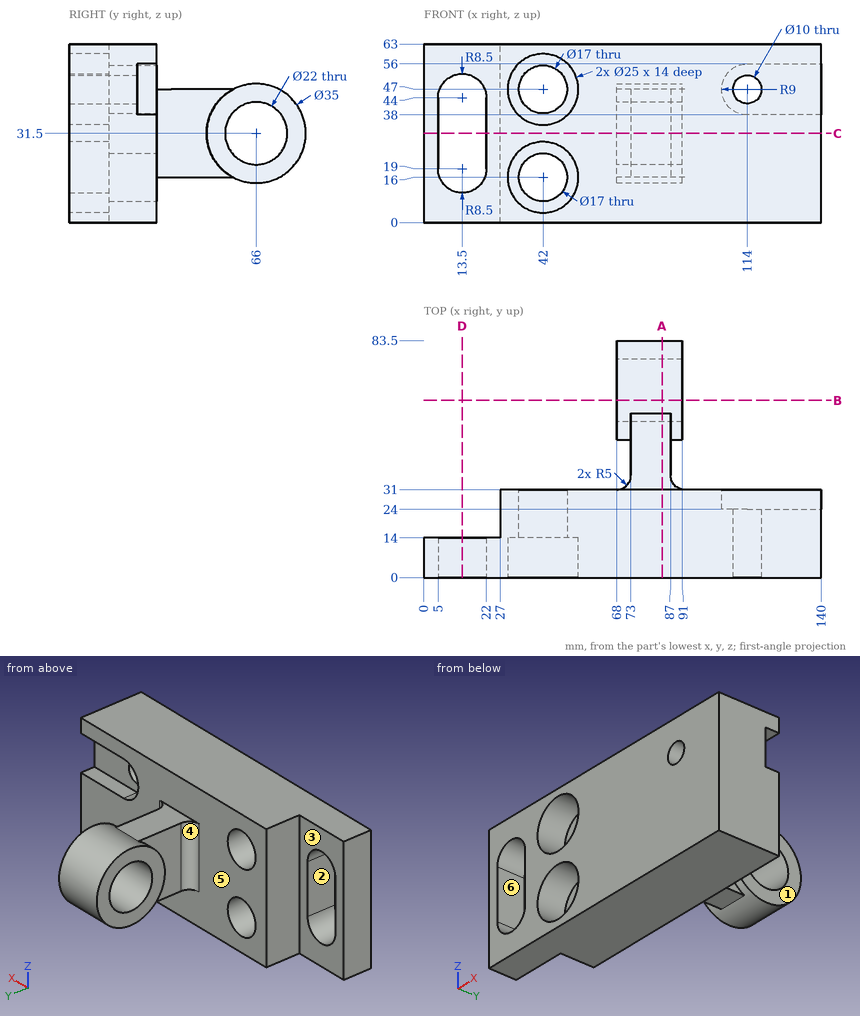
Here's the drawing with two shaded views (mm, measured from the low corner). I have some questions. A direction names the side the tool comes from. Give positions to 0.01 mm unless a question says otherwise; leave off trailing zeros. Loops run counter-clockwise (first coordinate to the right, second up) from the corner with the lowest first, then second, coordinate; pieces in that order, holes last. Notation, with made-up numbers: (-1, 32.25) - (30, 32.25) arc R17 cw to (30, 57.25) - close; hole circle Ø6 at (35, 40). An arc over 180 degrees is marked (long way). One line per item, written item: value.
(1) If we mould it in two halves opening along X, with no side actions, what happens to the marked faces 4, 5 and 6? For each: released by +X, released by -X, zero draft, split by the parting line, or undercut.
Verdict:
face 4: released by -X
face 5: zero draft
face 6: undercut
(2) On a 3-axis mill with a long thin cutter (end or side, diameter ignored), from which of +Z, -Z, +X, -X, +Y, -Y can I reach the whole of each face in a straight line? I mean the marked faces 1, 2 and 3. Say none if no direction works.
Verdict:
face 1: +Z, -Z, +X, +Y
face 2: +Y, -Y
face 3: +Z, -Z, -X, +Y
(3) I'm going to push flat-ended pins straight in: pin 1 (8 mm diameter, centred on y = 37, z = 46.5, fed in from -X); pin 2 (19 mm diameter, centred on x = 89, z = 44, fed in from +Y); pin 3 (17.5 mm diameter, centred on y = 50.5, z = 30.5, fed in from +X). Where does each tip first touch, or does it pass through?
Verdict:
pin 1: x = 72
pin 2: y = 83.24
pin 3: x = 91
(4) If we section it at B-B, the plane y = 62.5: List the corners of the cut face in (x, z) for me, plus the area to 3 significant figures.
Verdict:
outline: (68, 14.35) - (91, 14.35) - (91, 21.07) - (68, 21.07) - close; (68, 41.93) - (91, 41.93) - (91, 48.65) - (68, 48.65) - close
area: 309 mm^2
(5) If we section it at A-A, the plane x = 84: List the corners of the cut face in (y, z) for me.
Verdict:
outline: (0, 0) - (31, 0) - (31, 16) - (57.88, 16) arc R17.5 ccw (long way) to (57.88, 47) - (31, 47) - (31, 63) - (0, 63) - close; hole circle Ø22 at (66, 31.5)
(6) I need wall thicknesses on line 1 along Y through (x, z) = (74, 31); line 2 along X through (y, z) = (19.5, 16); line 3 along Z through (x, y) = (42, 22). Which ranges of each line are inside material? Lowest first, please.
Verdict:
line 1: 0 to 55.01, 76.99 to 83.49
line 2: 27 to 33.5, 50.5 to 140
line 3: 0 to 7.5, 24.5 to 38.5, 55.5 to 63
(7) If we section it at D-D, the plane x = 13.5: List the corners of the cut face in (y, z) for me, plus the area to 3 significant figures.
Verdict:
outline: (0, 0) - (14, 0) - (14, 10.5) - (0, 10.5) - close; (0, 52.5) - (14, 52.5) - (14, 63) - (0, 63) - close
area: 294 mm^2
(8) If we section it at C-C, the plane z = 31.5: List the corners of the cut face in (x, y) for me.
Verdict:
outline: (0, 0) - (5, 0) - (5, 14) - (0, 14) - close; (22, 0) - (140, 0) - (140, 31) - (92, 31) arc R5 cw to (87, 36) - (87, 48.5) - (91, 48.5) - (91, 55) - (68, 55) - (68, 48.5) - (73, 48.5) - (73, 36) arc R5 cw to (68, 31) - (27, 31) - (27, 14) - (22, 14) - close; (68, 77) - (91, 77) - (91, 83.5) - (68, 83.5) - close
